For this review, take the finished solid that the model builds, in its own axes (mm). Face numbers are marked on the shaded views. A direction names the side the tool comes from. Round coordinates to 2 decimals unless told otherwise and drop trailing zeros. Loops run counter-clockwise (first coordinate to the right, second up) from the corner with the lowest first, then second, coordinate; pieces in that order, holes last.
1. To check wall thickness, follow line 1 along Z through (x, y) = (17, -17) (3 decimals); line 2 along Y through (x, z) = (0, 1.3); line 3 along X through (y, z) = (17.5, 40). State the ranges of each line that lie inside material, in increasing order.
2. Consider section A-A on x = 0. State the section outline as (y, z) points (3 decimals).
3. Consider section D-D on z = 25.5. State the section outline as (x, y) points, then the cut area to 3 significant figures.
4. Tool access review of the marked faces 1 and 2: name each direction out of +Z, -Z, +X, -X, +Y, -Y from which nothing blocks a thin tool from reaching the whole face with its end or side.
5. Clearance check with a flat-ended pin moving along its axis: pin 1 Ø22 at (y, z) = (9.5, 35.5) entering from -X. State where the tip first meets the part, or that it passes through.
6. Consider section C-C on y = 9.5. State the section outline as (x, z) points (3 decimals).
from build123d import *

# Parameters (mm, degrees)
SKETCH1_W                    = 87.64016
SKETCH1_H                    = 44.27474
SKETCH1_R                    = 3
BASE_FLANGE1_DEPTH           = 3.175
EDGE_FLANGE2_STRIP_W         = 14.7
EDGE_FLANGE2_STRIP_H         = 3.175
EDGE_FLANGE2_STRIP_CUT_DEPTH = 44.27474
EDGE_FLANGE2_DEPTH           = 44.27474
CUT_EXTRUDE2_DEPTH           = 107.386542553
CUT_EXTRUDE2_DEPTH_BACK      = 3.175
M6_CLEARANCE_HOLE2_D         = 7
M6_CLEARANCE_HOLE2_DEPTH     = 3.175


# Sheet-metal steps are written as plain solids
with BuildPart() as part:
    # Sketch1 → Base-Flange1 (new body)
    with BuildSketch(Plane.XY):
        Rectangle(SKETCH1_W, SKETCH1_H)
        Circle(SKETCH1_R, mode=Mode.SUBTRACT)
    extrude(amount=BASE_FLANGE1_DEPTH)

    # Edge-Flange2 strip (across the edge) → Edge-Flange2 strip cut (cut)
    with BuildSketch(Plane(origin=(43.82008, -22.13737, 3.175), x_dir=(-1, 0, 0), z_dir=(0, 1, 0))):
        with Locations((-6.35, -1.5875)):
            Rectangle(EDGE_FLANGE2_STRIP_W, EDGE_FLANGE2_STRIP_H)
    extrude(amount=EDGE_FLANGE2_STRIP_CUT_DEPTH, mode=Mode.SUBTRACT)

    # Edge-Flange2 section (across the edge) → Edge-Flange2 (add)
    with BuildSketch(Plane(origin=(43.82008, -22.13737, 3.175), x_dir=(-1, 0, 0), z_dir=(0, 1, 0))):
        with BuildLine():
            Line((-3.175, 1), (-3.175, 47.625))
            Line((-3.175, 47.625), (0, 47.625))
            Line((0, 47.625), (0, 1))
            ThreePointArc((0, 1), (0.292893219, 0.292893219), (1, 0))
            Line((1, 0), (1, -3.175))
            ThreePointArc((1, -3.175), (-1.952170811, -1.952170811), (-3.175, 1))
        make_face()
    extrude(amount=EDGE_FLANGE2_DEPTH)

    # Sketch13 → Cut-Extrude2 (cut, two sides: drawn at the far end of the back side and taken through both)
    with BuildSketch(Plane(origin=(46.99508, 0, 0), x_dir=(0, 0, -1), z_dir=(1, 0, 0)).offset(-CUT_EXTRUDE2_DEPTH_BACK)):
        Polygon((-4.175, -22.13737), (-50.8, 22.13737), (-50.8, -22.13737), align=None)
    extrude(amount=CUT_EXTRUDE2_DEPTH + CUT_EXTRUDE2_DEPTH_BACK, mode=Mode.SUBTRACT)

    # M6 Clearance Hole2
    with Locations(Plane.XY.offset(3.175)):
        with Locations((0, 0)):
            Hole(M6_CLEARANCE_HOLE2_D / 2, depth=M6_CLEARANCE_HOLE2_DEPTH)


solid = part.part
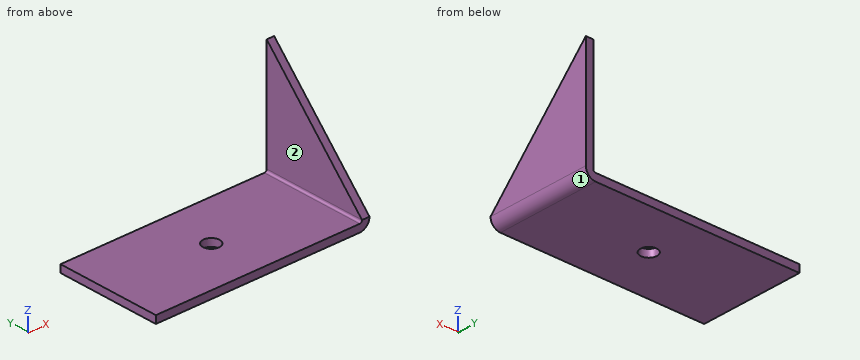
Resolved:
1. line 1: z = 0 to 3.175
1. line 2: y = -22.14 to -3.5, 3.5 to 22.14
1. line 3: x = 43.82 to 47
2. outline: (-22.137, 0) - (-3.5, 0) - (-3.5, 3.175) - (-22.137, 3.175) - close; (3.5, 0) - (22.137, 0) - (22.137, 3.175) - (3.5, 3.175) - close
3. outline: (43.82, -1.89) - (47, -1.89) - (47, 22.14) - (43.82, 22.14) - close
3. area: 76.3 mm2
4. face 1: -Z, +X, +Y, -Y
4. face 2: +Z, -X, +Y, -Y
5. pin 1: stops at x = 43.82
6. outline: (-43.82, 0) - (42.82, 0) arc R4.175 ccw to (46.995, 4.175) - (46.995, 37.492) - (43.82, 37.492) - (43.82, 4.175) arc R1 cw to (42.82, 3.175) - (-43.82, 3.175) - close
